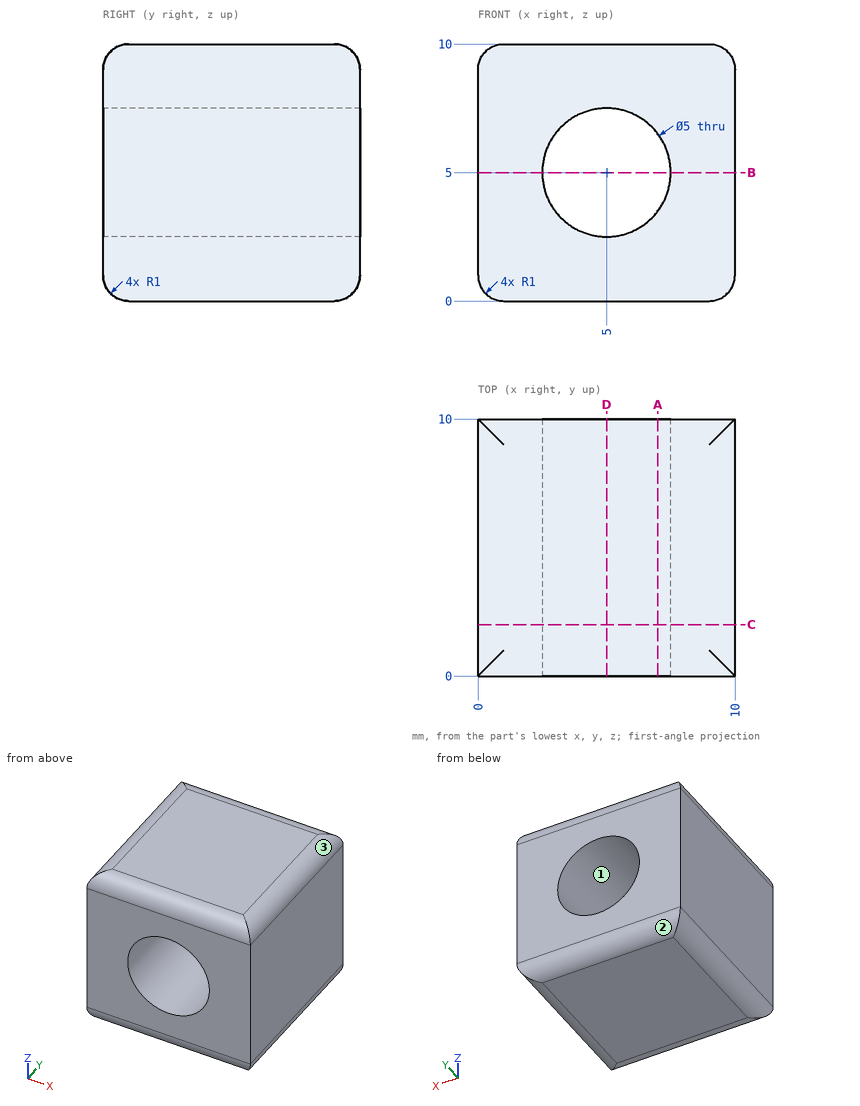
Could you check a few things on this drawing? It's one solid part, dimensions in mm from its lowest x, y, z. Round coordinates to 2 decimals unless told otherwise and drop trailing zeros. Loops run counter-clockwise (first coordinate to the right, second up) from the corner with the lowest first, then second, coordinate; pieces in that order, holes last.
Q1. I want a section at D-D (x = 5). Write out the boundary of the cut face in (y, z), and give its area (3 significant figures).
Q2. I want a section at B-B (z = 5). Write out the boundary of the cut face in (x, y).
Q3. I want a section at C-C (y = 2). Write out the boundary of the cut face in (x, z).
Q4. I want a section at A-A (x = 7). Write out the boundary of the cut face in (y, z), and give its area (3 significant figures).
Q5. Please list where these lines run through material, in increasing order: L1, parallel to Z at x = 5, y = 4.5; L2, parallel to Z at x = 3.75, y = 8.5; L3, parallel to X at y = 4.25, z = 5.25.
Q6. For P1, Ø3, axis at x = 5, z = 5, coming from the +Y side, with a flat end and sliding along its axis, tell me the tip position at first contact or that it passes through.
Q7. Thinking about a two-plate mould opening in X: for the marked faces 1, 2 and 3, which applies, pulls with the +X half, pulls with the -X half, needs draft (parallel to the pull), parting line crosses it, or undercut?
Answer below:
1. outline: (0, 1) arc R1 ccw to (1, 0) - (9, 0) arc R1 ccw to (10, 1) - (10, 2.5) - (0, 2.5) - close; (0, 7.5) - (10, 7.5) - (10, 9) arc R1 ccw to (9, 10) - (1, 10) arc R1 ccw to (0, 9) - close
1. area: 49.1 mm2
2. outline: (0, 0) - (2.5, 0) - (2.5, 10) - (0, 10) - close; (7.5, 0) - (10, 0) - (10, 10) - (7.5, 10) - close
3. outline: (0, 1) arc R1 ccw to (1, 0) - (9, 0) arc R1 ccw to (10, 1) - (10, 9) arc R1 ccw to (9, 10) - (1, 10) arc R1 ccw to (0, 9) - close; hole circle Ø5 at (5, 5)
4. outline: (0, 1) arc R1 ccw to (1, 0) - (9, 0) arc R1 ccw to (10, 1) - (10, 3.5) - (0, 3.5) - close; (0, 6.5) - (10, 6.5) - (10, 9) arc R1 ccw to (9, 10) - (1, 10) arc R1 ccw to (0, 9) - close
4. area: 69.1 mm2
5. L1: z = 0 to 2.5, 7.5 to 10
5. L2: z = 0 to 2.83, 7.17 to 10
5. L3: x = 0 to 2.51, 7.49 to 10
6. P1: passes through
7. face 1: undercut
7. face 2: needs draft
7. face 3: pulls with the +X half
